Here's how the part is built. I have some questions about the finished solid (model axes, mm). Face numbers are marked on the shaded views. A direction names the side the tool comes from. Round coordinates to 2 decimals unless told otherwise and drop trailing zeros. Order: outer loops, then holes, each group sorted by start corner. A loop starts at its lowest first (then second) coordinate and runs counter-clockwise, first axis right, second up.
```python
from build123d import *

# Parameters (mm, degrees)
BOSS_EXTRUDE1_DEPTH = 180
SKETCH12_R          = 1.55
CUT_EXTRUDE1_DEPTH  = 20
SKETCH13_R          = 2
CUT_EXTRUDE2_DEPTH  = 20


with BuildPart() as part:
    # Sketch1 → Boss-Extrude1 (new body)
    with BuildSketch(Plane.XZ):
        with BuildLine():
            Line((-17.8, -24.145), (-3.6, -24.145))
            Line((-3.6, -24.145), (3.6, -24.145))
            Line((3.6, -24.145), (17.8, -24.145))
            ThreePointArc((17.8, -24.145), (19.214213562, -23.559213562), (19.8, -22.145))
            Line((19.8, -22.145), (19.8, -18.345))
            ThreePointArc((19.8, -18.345), (20.385786438, -16.930786438), (21.8, -16.345))
            Line((21.8, -16.345), (23.4, -16.345))
            ThreePointArc((23.4, -16.345), (27, -12.745), (23.4, -9.145))
            Line((23.4, -9.145), (21.8, -9.145))
            ThreePointArc((21.8, -9.145), (20.385786438, -8.559213562), (19.8, -7.145))
            Line((19.8, -7.145), (19.8, 12.945))
            ThreePointArc((19.8, 12.945), (19.214213562, 14.359213562), (17.8, 14.945))
            Line((17.8, 14.945), (5.6, 14.945))
            ThreePointArc((5.6, 14.945), (4.185786438, 15.530786438), (3.6, 16.945))
            Line((3.6, 16.945), (3.6, 18.545))
            ThreePointArc((3.6, 18.545), (0, 22.145), (-3.6, 18.545))
            Line((-3.6, 18.545), (-3.6, 16.945))
            ThreePointArc((-3.6, 16.945), (-4.185786438, 15.530786438), (-5.6, 14.945))
            Line((-5.6, 14.945), (-17.8, 14.945))
            ThreePointArc((-17.8, 14.945), (-19.214213562, 14.359213562), (-19.8, 12.945))
            Line((-19.8, 12.945), (-19.8, -7.145))
            ThreePointArc((-19.8, -7.145), (-20.385786438, -8.559213562), (-21.8, -9.145))
            Line((-21.8, -9.145), (-23.4, -9.145))
            ThreePointArc((-23.4, -9.145), (-27, -12.745), (-23.4, -16.345))
            Line((-23.4, -16.345), (-21.8, -16.345))
            ThreePointArc((-21.8, -16.345), (-20.385786438, -16.930786438), (-19.8, -18.345))
            Line((-19.8, -18.345), (-19.8, -22.145))
            ThreePointArc((-19.8, -22.145), (-19.214213562, -23.559213562), (-17.8, -24.145))
        make_face()
    extrude(amount=-BOSS_EXTRUDE1_DEPTH)

    # Sketch12 → Cut-Extrude1 (cut)
    with BuildSketch(Plane.XZ):
        with Locations(Location((0, 18.545, 0), (0, 0, 270))):
            Circle(SKETCH12_R)
        with Locations(Location((-23.4, -12.745, 0), (0, 0, 270))):
            Circle(SKETCH12_R)
        with Locations(Location((23.4, -12.745, 0), (0, 0, 270))):
            Circle(SKETCH12_R)
    extrude(amount=-CUT_EXTRUDE1_DEPTH, mode=Mode.SUBTRACT)

    # Sketch13 → Cut-Extrude2 (cut)
    with BuildSketch(Plane(origin=(0, 180, 0), x_dir=(1, 0, 0), z_dir=(0, 1, 0))):
        with Locations(Location((0, 12.745, 0), (0, 0, 270))):
            Circle(SKETCH13_R)
        with Locations(Location((10, -7.255, 0), (0, 0, 270))):
            Circle(SKETCH13_R)
        with Locations(Location((-10, -7.255, 0), (0, 0, 90))):
            Circle(SKETCH13_R)
    extrude(amount=-CUT_EXTRUDE2_DEPTH, mode=Mode.SUBTRACT)


solid = part.part
```
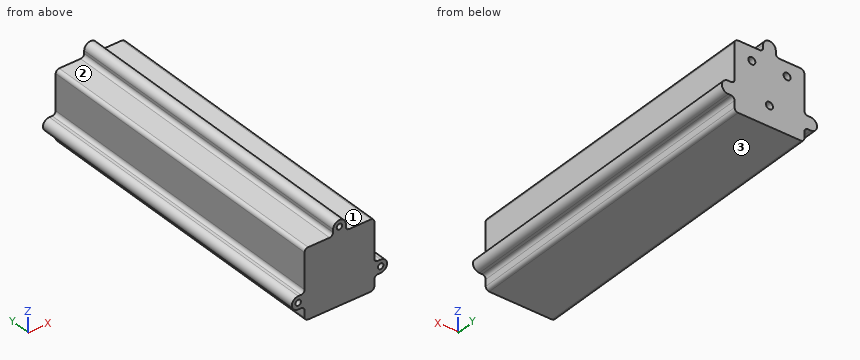
1. I need wall thicknesses on probe 1 along X at (y, z) = (139.5, -12.5); probe 2 along X at (y, z) = (110, -16); probe 3 along Z at (x, y) = (-17, 154) (3 decimals). Which ranges of each line are inside material? Lowest first, please.
Evaluation:
probe 1: x = -26.99 to 26.99
probe 2: x = -24.94 to 24.94
probe 3: z = -24.145 to 14.945
2. I'm going to push flat-ended pins straight in: P1, Ø22, axis at y = 80.5, z = 1, coming from the +X side; P2, Ø6, axis at y = 71.5, z = 16.5, coming from the -X side; P3, Ø4, axis at y = 81, z = -21, coming from the -X side. Where does each tip first touch, or does it pass through?
Evaluation:
P1: stops at x = 25.73
P2: stops at x = -19.72
P3: stops at x = -19.8
3. If we section it at C-C, the plane y = 49: Write out the boundary of the cut face in (x, z) (3 decimals).
Evaluation:
outline: (-23.4, -16.345) - (-21.8, -16.345) arc R2 cw to (-19.8, -18.345) - (-19.8, -22.145) arc R2 ccw to (-17.8, -24.145) - (17.8, -24.145) arc R2 ccw to (19.8, -22.145) - (19.8, -18.345) arc R2 cw to (21.8, -16.345) - (23.4, -16.345) arc R3.6 ccw to (23.4, -9.145) - (21.8, -9.145) arc R2 cw to (19.8, -7.145) - (19.8, 12.945) arc R2 ccw to (17.8, 14.945) - (5.6, 14.945) arc R2 cw to (3.6, 16.945) - (3.6, 18.545) arc R3.6 ccw to (-3.6, 18.545) - (-3.6, 16.945) arc R2 cw to (-5.6, 14.945) - (-17.8, 14.945) arc R2 ccw to (-19.8, 12.945) - (-19.8, -7.145) arc R2 cw to (-21.8, -9.145) - (-23.4, -9.145) arc R3.6 ccw to start
4. If we section it at D-D, the plane z = 1.5: Write out the boundary of the cut face in (x, y), and give its area (3 significant figures).
Evaluation:
outline: (-19.8, 0) - (19.8, 0) - (19.8, 180) - (-19.8, 180) - close
area: 7,130 mm2
5. If we section it at B-B, the plane x = -10: Write out the boundary of the cut face in (y, z) (3 decimals).
Evaluation:
outline: (0, -24.145) - (180, -24.145) - (180, 5.255) - (160, 5.255) - (160, 9.255) - (180, 9.255) - (180, 14.945) - (0, 14.945) - close
6. On a 3-axis mill with a long thin cutter (end or side, diameter ignored), from which of +Z, -Z, +X, -X, +Y, -Y can I reach the whole of each face in a straight line? I mean the marked faces 1, 2 and 3. Say none if no direction works.
Evaluation:
face 1: +Z, +X, +Y, -Y
face 2: +Z, -X, +Y, -Y
face 3: -Z, +X, -X, +Y, -Y
7. If we section it at A-A, the plane y = 168.5: State how many separate pieces and enclosed holes the cut face has, and give its area (3 significant figures).
Evaluation:
separate pieces: 1
enclosed holes: 3
area: 1,650 mm2
